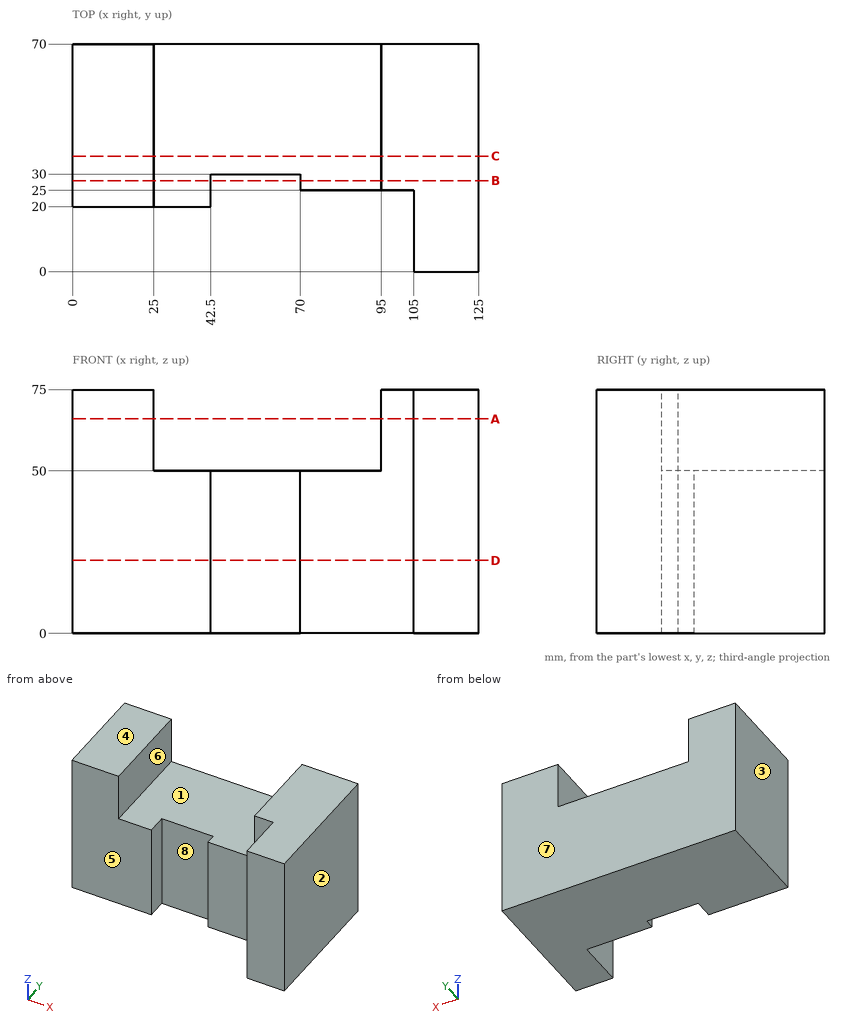
Print and shaded views of the part. All mm, measured from the part's lowest x, y and z. A direction names the side the tool comes from. Round coordinates to 2 decimals unless told otherwise and drop trailing zeros. Write each loop counter-clockwise with the first axis right and the second up, starting at its lowest first coordinate (ties: lowest second). Pieces come first, ordered by that corner, then holes. Notation, with made-up numbers: (36, -34) -> (94, -34) arc R35 ccw to (94, 2) -> close; hole circle Ø4 at (-0.75, 34). An arc over 180 degrees is marked (long way). Answer in a Markdown table with one row per item. Add a question column.
Item 1: Which spindle directions (+Z, -Z, +X, -X, +Y, -Y) get a long thin tool onto all of the face, cutting with end or side? Do the marked faces 5, 6, 7 and 8. Say none if no direction does.
Item 2: Saw through at D-D, the plane z = 22.5. Write the cut outline in (x, y).
Item 3: Saw through at B-B, the plane y = 28. Write the cut outline in (x, z).
Item 4: Mould opens along X. For the marked faces 1, 2, 3 and 4 say: pulls with the +X half, pulls with the -X half, needs draft (parallel to the pull), parting line crosses it, or undercut.
Item 5: Saw through at A-A, the plane z = 66. Write the cut outline in (x, y), then the cut area to 3 significant figures.
Item 6: Drop flat-ended pins along their axis: pin 1 Ø3 at (y, z) = (10.5, 17) entering from -X; pin 2 Ø6 at (x, z) = (18, 13.5) entering from -Y; pin 3 Ø14 at (x, z) = (53, 28) entering from -Y; pin 4 Ø1.5 at (x, y) = (41.5, 19) entering from +Z. Give the stop position or say it passes through.
Item 7: Drill centre lines: line 1 (X direction, y = 22, z = 51.5); line 2 (X direction, y = 65.5, z = 61.5); line 3 (Y direction, x = 101, z = 71). Where is each one in solid material? Low to high. Write a range as from..to.
Item 8: Saw through at C-C, the plane y = 35.5. Write the cut outline in (x, z), then the cut area to 4 significant figures.
Findings below:
| question | item | result |
|---|---|---|
| 1 | face 5 | +Z, -Z, -X, -Y |
| 1 | face 6 | +Z, +Y, -Y |
| 1 | face 7 | +Z, -Z, +X, -X, +Y |
| 1 | face 8 | +Z, -Z, -Y |
| 2 | outline | (0, 20) -> (42.5, 20) -> (42.5, 30) -> (70, 30) -> (70, 25) -> (105, 25) -> (105, 0) -> (125, 0) -> (125, 70) -> (0, 70) -> close |
| 3 | outline | (0, 0) -> (42.5, 0) -> (42.5, 50) -> (25, 50) -> (25, 75) -> (0, 75) -> close; (70, 0) -> (125, 0) -> (125, 75) -> (95, 75) -> (95, 50) -> (70, 50) -> close |
| 4 | face 1 | undercut |
| 4 | face 2 | pulls with the +X half |
| 4 | face 3 | pulls with the -X half |
| 4 | face 4 | needs draft |
| 5 | outline | (0, 20) -> (25, 20) -> (25, 70) -> (0, 70) -> close; (95, 25) -> (105, 25) -> (105, 0) -> (125, 0) -> (125, 70) -> (95, 70) -> close |
| 5 | area | 3,100 mm^2 |
| 6 | pin 1 | stops at x = 105 |
| 6 | pin 2 | stops at y = 20 |
| 6 | pin 3 | stops at y = 30 |
| 6 | pin 4 | passes through |
| 7 | line 1 | x = 0..25, 105..125 |
| 7 | line 2 | x = 0..25, 95..125 |
| 7 | line 3 | y = 25..70 |
| 8 | outline | (0, 0) -> (125, 0) -> (125, 75) -> (95, 75) -> (95, 50) -> (25, 50) -> (25, 75) -> (0, 75) -> close |
| 8 | area | 7,625 mm^2 |
